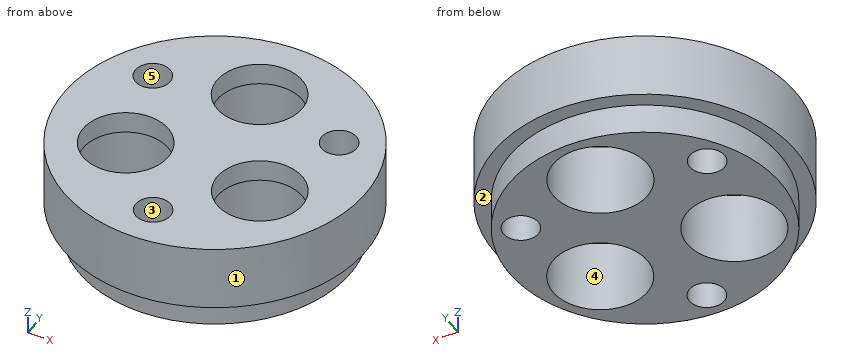
from build123d import *

# Parameters (mm, degrees)
ESQUISSE1_R             = 34.5
BOSS_EXTRU_1_DEPTH      = 15
ESQUISSE2_R             = 10.8
ENL_V_MAT_EXTRU_1_DEPTH = 15
ESQUISSE3_R             = 11
ESQUISSE3_R_2           = 9.75
BOSS_EXTRU_2_DEPTH      = 5
ESQUISSE4_R             = 4
ENL_V_MAT_EXTRU_2_DEPTH = 52.044098582
ESQUISSE6_R             = 31
ESQUISSE6_R_2           = 4
ESQUISSE6_R_3           = 10.8
BOSS_EXTRU_5_DEPTH      = 7


with BuildPart() as part:
    # Esquisse1 → Boss.-Extru.1 (new body)
    with BuildSketch(Plane.XY):
        Circle(ESQUISSE1_R)
    extrude(amount=BOSS_EXTRU_1_DEPTH)

    # Esquisse2 → Enlèv. mat.-Extru.1 (cut)
    with BuildSketch(Plane.XY.offset(15)):
        with Locations((0, 18)):
            Circle(ESQUISSE2_R)
        with Locations((15.588457268, -9)):
            Circle(ESQUISSE2_R)
        with Locations((-15.588457268, -9)):
            Circle(ESQUISSE2_R)
    extrude(amount=-ENL_V_MAT_EXTRU_1_DEPTH, mode=Mode.SUBTRACT)

    # Esquisse3 → Boss.-Extru.2 (add)
    # profile 1 of 3: a face of its own
    with BuildSketch(Plane.XY.offset(15)):
        with Locations((0, 18)):
            Circle(ESQUISSE3_R)
        with Locations((0, 18)):
            Circle(ESQUISSE3_R_2, mode=Mode.SUBTRACT)
    # profile 2 of 3: a face of its own
    with BuildSketch(Plane.XY.offset(15)):
        with Locations((15.588457268, -9)):
            Circle(ESQUISSE3_R)
        with Locations((15.588457268, -9)):
            Circle(ESQUISSE3_R_2, mode=Mode.SUBTRACT)
    # profile 3 of 3: a face of its own
    with BuildSketch(Plane.XY.offset(15)):
        with Locations((-15.588457268, -9)):
            Circle(ESQUISSE3_R)
        with Locations((-15.588457268, -9)):
            Circle(ESQUISSE3_R_2, mode=Mode.SUBTRACT)
    extrude(amount=-BOSS_EXTRU_2_DEPTH)

    # Esquisse4 → Enlèv. mat.-Extru.2 (cut, through all)
    with BuildSketch(Plane.XY.offset(15)):
        with Locations((21.650635095, 12.5)):
            Circle(ESQUISSE4_R)
        with Locations((-21.650635095, 12.5)):
            Circle(ESQUISSE4_R)
        with Locations((0, -25)):
            Circle(ESQUISSE4_R)
    extrude(amount=-ENL_V_MAT_EXTRU_2_DEPTH, mode=Mode.SUBTRACT)

    # Esquisse6 → Boss.-Extru.5 (add)
    with BuildSketch(Plane(origin=(0, 0, 0), x_dir=(-1, 0, 0), z_dir=(0, 0, -1))):
        Circle(ESQUISSE6_R)
        with Locations(Location((0, -25, 0), (0, 0, 180))):
            Circle(ESQUISSE6_R_2, mode=Mode.SUBTRACT)
        with Locations(Location((-15.588457268, -9, 0), (0, 0, 180))):
            Circle(ESQUISSE6_R_3, mode=Mode.SUBTRACT)
        with Locations(Location((0, 18, 0), (0, 0, 180))):
            Circle(ESQUISSE6_R_3, mode=Mode.SUBTRACT)
        with Locations(Location((15.588457268, -9, 0), (0, 0, 180))):
            Circle(ESQUISSE6_R_3, mode=Mode.SUBTRACT)
        with Locations(Location((21.650635095, 12.5, 0), (0, 0, 180))):
            Circle(ESQUISSE6_R_2, mode=Mode.SUBTRACT)
        with Locations(Location((-21.650635095, 12.5, 0), (0, 0, 180))):
            Circle(ESQUISSE6_R_2, mode=Mode.SUBTRACT)
    extrude(amount=BOSS_EXTRU_5_DEPTH)


solid = part.part
Could you check a few things on this model? Use its own coordinates, in mm. Face numbers are marked on the shaded views. A direction names the side the tool comes from. Round coordinates to 2 decimals unless told otherwise and drop trailing zeros. Write each loop counter-clockwise with the first axis right and the second up, starting at its lowest first coordinate (ties: lowest second). Pieces come first, ordered by that corner, then holes. Notation, with made-up numbers: (15.5, 12) - (40.5, 12) arc R21 cw to (40.5, 44) - close; hole circle Ø6 at (-7.75, 84). An arc over 180 degrees is marked (long way). Use a Markdown table: item, result.
Q1. Please list where these lines run through material, in increasing order: L1, parallel to X at y = -14.5, z = 6; L2, parallel to Y at x = 1, z = 13; L3, parallel to Y at x = -8.5, z = 6.25.
Output values:
| item | result |
|---|---|
| L1 | -31.3 to -24.88, -6.29 to 6.29, 24.88 to 31.3 |
| L2 | -34.49 to -28.87, -21.13 to 8.3, 27.7 to 34.49 |
| L3 | -33.44 to -17.15, -0.85 to 11.34, 24.66 to 33.44 |
Q2. For pin 1 (12 mm diameter, centred on x = 7.5, y = 24.5, fed in from -Z); pin 2 (8 mm diameter, centred on x = -7, z = 0, fed in from +Y); pin 3 (5 mm diameter, centred on y = -8.5, z = 5, fed in from +X); pin 4 (6 mm diameter, centred on x = 13.5, z = 4, fed in from +Y), each with a flat end and sliding along its axis, tell me the tip position at first contact or that it passes through.
Output values:
| item | result |
|---|---|
| pin 1 | z = -7 |
| pin 2 | y = 34.37 |
| pin 3 | x = 33.97 |
| pin 4 | y = 32.86 |
Q3. I want a section at D-D (y = 18). List the corners of the cut face in (x, z) for me.
Output values:
| item | result |
|---|---|
| outline | (-29.43, 0) - (-25.24, 0) - (-25.24, -7) - (-10.8, -7) - (-10.8, 10) - (-9.75, 10) - (-9.75, 15) - (-29.43, 15) - close; (9.75, 10) - (10.8, 10) - (10.8, -7) - (25.24, -7) - (25.24, 0) - (29.43, 0) - (29.43, 15) - (9.75, 15) - close |
Q4. I want a section at B-B (x = 0). List the corners of the cut face in (y, z) for me.
Output values:
| item | result |
|---|---|
| outline | (-34.5, 0) - (-31, 0) - (-31, -7) - (-29, -7) - (-29, 15) - (-34.5, 15) - close; (-21, -7) - (7.2, -7) - (7.2, 10) - (8.25, 10) - (8.25, 15) - (-21, 15) - close; (27.75, 10) - (28.8, 10) - (28.8, -7) - (31, -7) - (31, 0) - (34.5, 0) - (34.5, 15) - (27.75, 15) - close |
Q5. I want a section at C-C (y = -7). List the corners of the cut face in (x, z) for me.
Output values:
| item | result |
|---|---|
| outline | (-33.78, 0) - (-30.2, 0) - (-30.2, -7) - (-26.2, -7) - (-26.2, 10) - (-25.13, 10) - (-25.13, 15) - (-33.78, 15) - close; (-6.05, 10) - (-4.98, 10) - (-4.98, -7) - (4.98, -7) - (4.98, 10) - (6.05, 10) - (6.05, 15) - (-6.05, 15) - close; (25.13, 10) - (26.2, 10) - (26.2, -7) - (30.2, -7) - (30.2, 0) - (33.78, 0) - (33.78, 15) - (25.13, 15) - close |
Q6. Thinking about a two-plate mould opening in Y: for the marked faces 1, 2 and 3, which applies, released by +Y, released by -Y, zero draft, split by the parting line, or undercut?
Output values:
| item | result |
|---|---|
| face 1 | split by the parting line |
| face 2 | zero draft |
| face 3 | undercut |
Q7. I want a section at A-A (z = 11.25). List the corners of the cut face in (x, y) for me.
Output values:
| item | result |
|---|---|
| outline | circle Ø69 at (0, 0); hole circle Ø8 at (-21.65, 12.5); hole circle Ø19.5 at (-15.59, -9); hole circle Ø19.5 at (0, 18); hole circle Ø8 at (0, -25); hole circle Ø19.5 at (15.59, -9); hole circle Ø8 at (21.65, 12.5) |
Q8. For the marked faces 4 and 5, which set-ups out of +Z, -Z, +X, -X, +Y, -Y let a thin tool reach every point of the face, with its end or its side?
Output values:
| item | result |
|---|---|
| face 4 | -Z |
| face 5 | +Z, -Z |
